```python
from build123d import *

# Parameters (mm, degrees)
F1_DEPTH = 1


# Not quite as in the source:
# - a feature names something its author has since deleted; it is built from what else it names


with BuildPart() as f1:
    # F0 (on Top) → F1 (new body)
    with BuildSketch(Plane.XY):
        with BuildLine():
            add(Edge.make_bspline(
                [(-16.6099965572, 10.2172633633), (-15.4212118205, 9.5285409053), (-12.9551826674, 8.0998468723), (-7.766656534, 7.5933629956), (-6.3511176621, 8.4439850217), (-5.7889274321, 8.7818149477)],
                knots=[0, 0, 0, 0, 0.3594226743, 0.7455906573, 1, 1, 1, 1], degree=3))
            add(Edge.make_bspline(
                [(-16.6099965572, 10.2172633633), (-16.3713958805, 9.4307097449), (-15.904194945, 7.8905691575), (-15.5435341339, 6.4249386215), (-15.3670636937, 5.7078092359)],
                knots=[0, 0, 0, 0, 0.5107024806, 1, 1, 1, 1], degree=3))
            add(Edge.make_bspline(
                [(-22.5439389952, 13.8567826848), (-20.9328268461, 12.3755889493), (-17.8750260099, 9.497072632), (-16.1981091624, 6.9589873468), (-15.3670636937, 5.7078092359)],
                knots=[0.1092468408, 0.1092468408, 0.1092468408, 0.1092468408, 0.5599397099, 1, 1, 1, 1], degree=3))
            add(Edge.make_bspline(
                [(-24.9835465397, 15.6512659715), (-24.5105414607, 15.2932659882), (-23.6115055046, 14.644329683), (-22.8821580713, 14.1081462449), (-22.5439389952, 13.8567826848)],
                knots=[0, 0, 0, 0, 0.5340013105, 1, 1, 1, 1], degree=3))
            add(Edge.make_bspline(
                [(-31.6534787416, 22.3535578698), (-31.4894436188, 21.7239753561), (-31.1336922454, 20.3585675093), (-29.1441485457, 18.4393483759), (-26.688509429, 16.66011353), (-24.9835465397, 15.6512659715)],
                knots=[0, 0, 0, 0, 0.1581489893, 0.342985814, 0.5895394489, 0.5895394489, 0.5895394489, 0.5895394489], degree=3))
            Line((-31.6534787416, 22.3535578698), (-31.3492268324, 22.8967126459))
            add(Edge.make_bspline(
                [(-34.7586423159, 29.0321223438), (-34.3418990536, 28.1776650529), (-33.5153831208, 26.4830424187), (-32.2770591236, 23.9047003589), (-31.6167279276, 23.1873231579), (-31.3492268324, 22.8967126459)],
                knots=[0, 0, 0, 0, 0.3769541602, 0.747603255, 1, 1, 1, 1], degree=3))
            add(Edge.make_bspline(
                [(-34.7586423159, 29.0321223438), (-35.5677944518, 27.4079633385), (-37.3288786405, 23.8782557478), (-37.627728367, 15.760880925), (-35.454224769, 11.2387606607), (-34.3599178116, 9.002301842)],
                knots=[0, 0, 0, 0, 0.3007790413, 0.6538294353, 1, 1, 1, 1], degree=3))
            add(Edge.make_bspline(
                [(-34.3599178116, 9.002301842), (-34.4460411955, 10.0396901503), (-34.5463298451, 11.768741471), (-34.4792390008, 13.4920788706), (-34.4357995181, 14.1820461029)],
                knots=[0, 0, 0, 0, 0.5004169403, 0.8340605609, 0.8340605609, 0.8340605609, 0.8340605609], degree=3))
            add(Edge.make_bspline(
                [(-18.5956805944, 0.7639901596), (-18.754914474, 1.762296212), (-19.1182465354, 4.0401820297), (-22.8890828074, 7.5134991963), (-26.9671489576, 11.505197563), (-29.4215545254, 13.182958406), (-32.0236221513, 14.6651885876), (-33.3319524476, 14.6676349212), (-34.0719301846, 14.3425994686), (-34.4357995181, 14.1820461029)],
                knots=[0, 0, 0, 0, 0.1460617246, 0.3332764838, 0.5324015784, 0.6782952182, 0.8179917645, 0.9100820113, 0.9991741954, 0.9991741954, 0.9991741954, 0.9991741954], degree=3))
            add(Edge.make_bspline(
                [(-23.1238305569, 1.4212612296), (-22.2308115866, 1.302547656), (-20.5628255796, 1.0808137554), (-19.2197091749, 0.8644946878), (-18.5956805944, 0.7639901596)],
                knots=[0, 0, 0, 0, 0.5353875671, 1, 1, 1, 1], degree=3))
            add(Edge.make_bspline(
                [(-23.1238305569, -10.3354090825), (-21.9181343668, -9.5672404628), (-19.5647077627, -8.0678341604), (-18.0730916869, -3.6305347437), (-21.2811829424, -0.4217720451), (-23.1238305569, 1.4212612296)],
                knots=[0, 0, 0, 0, 0.3089727792, 0.603091197, 1, 1, 1, 1], degree=3))
            add(Edge.make_bspline(
                [(-4.8519154079, -16.1593034863), (-7.4154305721, -15.6333116353), (-12.4370011009, -14.6029665784), (-19.2999839188, -12.0288214544), (-21.9779293524, -10.8428779902), (-23.1238305569, -10.3354090825)],
                knots=[0, 0, 0, 0, 0.3736855161, 0.7319980787, 1, 1, 1, 1], degree=3))
            add(Edge.make_bspline(
                [(-14.8473009467, -8.831509389), (-14.0171136981, -9.7171202904), (-12.2176917006, -11.6366724638), (-7.9071133303, -14.7016545165), (-5.7918028227, -15.7108788812), (-4.8519154079, -16.1593034863)],
                knots=[0, 0, 0, 0, 0.322473213, 0.6989572463, 1, 1, 1, 1], degree=3))
            add(Edge.make_bspline(
                [(-8.0227525905, -10.816199705), (-8.7445347825, -10.3543101709), (-10.2936553467, -9.3629826161), (-14.0342744282, -8.7559960985), (-14.6547502449, -8.8136254249), (-14.8473009467, -8.831509389)],
                knots=[0, 0, 0, 0, 0.3756557433, 0.806248815, 1, 1, 1, 1], degree=3))
            Line((-8.0227525905, -10.816199705), (-11.5278782323, -10.9786894172))
            add(Edge.make_bspline(
                [(-1.2948540742, -16.8027080712), (-4.3131749279, -15.2063237418), (-9.020596995, -12.7165640866), (-10.8657693402, -11.4376176997), (-11.5278782323, -10.9786894172)],
                knots=[4.22789e-05, 4.22789e-05, 4.22789e-05, 4.22789e-05, 0.6411820822, 1, 1, 1, 1], degree=3))
            add(Edge.make_bspline(
                [(-9.9178981036, -17.0243084431), (-8.0369774486, -17.152822121), (-4.8078227744, -17.3734537264), (-1.2910580124, -16.912451153), (-1.2927963607, -16.8091016917), (-1.2948540742, -16.8027080712)],
                knots=[0, 0, 0, 0, 0.5593319314, 0.960258114, 0.9872401448, 0.9872401448, 0.9872401448, 0.9872401448], degree=3))
            add(Edge.make_bspline(
                [(56.0104735196, -28.554501012), (51.9388012895, -30.6732939687), (43.1626287248, -35.2401872663), (23.7757696907, -34.1342565116), (6.1000439104, -28.3431760834), (-4.5392052922, -20.825090838), (-9.9178981036, -17.0243084431)],
                knots=[0, 0, 0, 0, 0.2229662615, 0.4805864215, 0.7374094706, 1, 1, 1, 1], degree=3))
            add(Edge.make_bspline(
                [(28.0218664557, -24.0996014327), (34.8843220952, -26.1370758676), (46.4307325782, -29.5652242463), (53.2458361821, -28.8461877297), (56.0104735196, -28.554501012)],
                knots=[0, 0, 0, 0, 0.5943367118, 1, 1, 1, 1], degree=3))
            Line((28.0218664557, -24.0996014327), (31.7761152983, -28.129896149))
            add(Edge.make_bspline(
                [(10.4167964309, -20.7992941141), (13.3020900166, -22.350921559), (18.7887841643, -25.301506991), (26.4258501352, -27.584558387), (30.1169773998, -27.9607848021), (31.7761152983, -28.129896149)],
                knots=[0, 0, 0, 0, 0.3791070825, 0.7209126382, 1, 1, 1, 1], degree=3))
            Line((10.4167964309, -20.7992941141), (13.8279302046, -21.5669311583))
            add(Edge.make_bspline(
                [(27.6213772595, -26.1221751571), (23.6067244924, -25.076781429), (17.2832552929, -23.4301844692), (14.7521015867, -22.0652823535), (13.8279302046, -21.5669311583)],
                knots=[0, 0, 0, 0, 0.6348813666, 1, 1, 1, 1], degree=3))
            add(Edge.make_bspline(
                [(10.8465477824, -10.9871085733), (13.7292478088, -14.2236435187), (19.1884297009, -20.3529087233), (24.9175139429, -24.2723702383), (27.6213772595, -26.1221751571)],
                knots=[0, 0, 0, 0, 0.5280461584, 1, 1, 1, 1], degree=3))
            Line((10.8465477824, -10.9871085733), (12.0913498104, -16.3664314896))
            add(Edge.make_bspline(
                [(-3.3141928725, -6.6230124794), (-1.2243299559, -8.513743245), (3.1043671989, -12.4299813966), (9.0277383612, -15.0245179581), (12.0913498104, -16.3664314896)],
                knots=[0, 0, 0, 0, 0.4827925914, 1, 1, 1, 1], degree=3))
            Line((-3.3141928725, -6.6230124794), (-1.909304643, -6.6230124794))
            add(Edge.make_bspline(
                [(10.2238217369, -14.115748927), (7.8172960071, -13.0456945157), (3.181551384, -10.9844246435), (-0.2561811543, -8.0392679882), (-1.909304643, -6.6230124794)],
                knots=[0, 0, 0, 0, 0.5191238788, 1, 1, 1, 1], degree=3))
            add(Edge.make_bspline(
                [(-0.9440209251, 3.5210286733), (1.0464920899, -0.3056682218), (4.6957007503, -7.3211538505), (8.4963093931, -11.9924692639), (10.2238217369, -14.115748927)],
                knots=[0, 0, 0, 0, 0.5454642911, 1, 1, 1, 1], degree=3))
            Line((-0.9440209251, 3.5210286733), (-0.6881441002, -2.2778437083))
            Line((-0.6881441002, -2.2778437083), (-7.6660518534, 2.0532717463))
            Line((-7.6660518534, 2.0532717463), (-7.6660518534, -0.5485964357))
            add(Edge.make_bspline(
                [(-9.6535952762, 4.4754715636), (-9.4700688508, 3.6180804257), (-9.0971451505, 1.8758709595), (-8.1480633424, 0.2679968231), (-7.6660518534, -0.5485964357)],
                knots=[0, 0, 0, 0, 0.4921286186, 1, 1, 1, 1], degree=3))
            Line((-9.6535952762, 4.4754715636), (-1.648212783, -0.4933868768))
            Line((-1.648212783, -0.4933868768), (-5.7889274321, 8.7818149477))
        make_face()
    extrude(amount=F1_DEPTH)


solid = f1.part
```
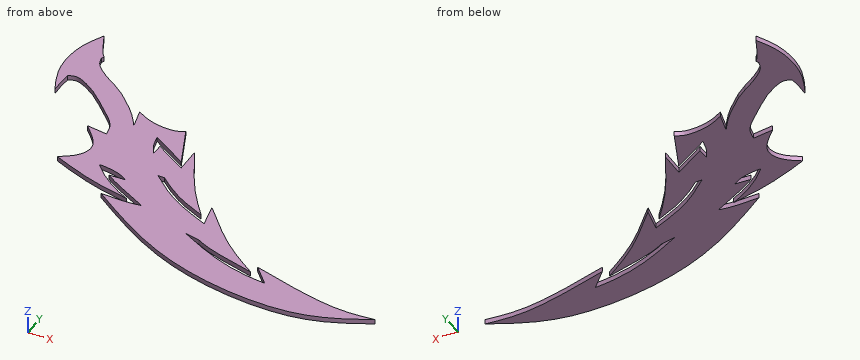
Can you work these out from the model? Positions are in its coordinate system, mm. Round coordinates to 2 decimals unless told otherwise and drop trailing zeros.
Item 1: Will this pin go through, and if not, where does the flat tip stop? pin 1 Ø5 at (x, y) = (12.5, -9.5) entering from -Z.
Item 2: Suppose I cut it at A-A, the plane y = -12.5. State how many separate pieces and enclosed holes the cut face has, then the cut area to 3 significant figures.
Item 3: Please list where these lines run through material, in increasing order: L1, parallel to Y at x = -21, z = 0.8; L2, parallel to Y at x = -20.5, z = 0.9; L3, parallel to X at y = -10.5, z = 0.55.
Reported:
1. pin 1: stops at z = 0
2. separate pieces: 4
2. enclosed holes: 0
2. area: 23.6 mm2
3. L1: y = -11.26 to -8.86, -0.79 to 1.13, 5.71 to 12.42
3. L2: y = -11.48 to -8.41, -1.38 to 1.06, 5.17 to 11.94
3. L3: x = -22.75 to -13.23, -8.52 to 1.22, 3.06 to 7.35
